```python
from build123d import *

# Parameters (mm, degrees)
F0_R     = 3.375
F0_R_2   = 2.6
F1_DEPTH = 13
F2_SIZE  = 3.5
F3_R     = 9
F4_DEPTH = 1.5


with BuildPart() as f1:
    # F0 (on Top) → F1 (new body)
    with BuildSketch(Plane.XY):
        with BuildLine():
            Line((-52.5, -62.5), (52.5, -62.5))
            ThreePointArc((52.5, -62.5), (59.571068, -59.571068), (62.5, -52.5))
            Line((62.5, -52.5), (62.5, 52.5))
            ThreePointArc((62.5, 52.5), (59.571068, 59.571068), (52.5, 62.5))
            Line((52.5, 62.5), (-52.5, 62.5))
            ThreePointArc((-52.5, 62.5), (-59.571068, 59.571068), (-62.5, 52.5))
            Line((-62.5, 52.5), (-62.5, -52.5))
            ThreePointArc((-62.5, -52.5), (-59.571068, -59.571068), (-52.5, -62.5))
        make_face()
        with Locations((-50, -50)):
            Circle(F0_R, mode=Mode.SUBTRACT)
        with Locations((-25, -50)):
            Circle(F0_R, mode=Mode.SUBTRACT)
        with Locations((0, -50)):
            Circle(F0_R, mode=Mode.SUBTRACT)
        with Locations((-50.3, -30)):
            Circle(F0_R_2, mode=Mode.SUBTRACT)
        with Locations((-25, -25)):
            Circle(F0_R, mode=Mode.SUBTRACT)
        with Locations((0, -25)):
            Circle(F0_R, mode=Mode.SUBTRACT)
        with Locations((25, -50)):
            Circle(F0_R, mode=Mode.SUBTRACT)
        with Locations((50, -50)):
            Circle(F0_R, mode=Mode.SUBTRACT)
        with Locations((25, -25)):
            Circle(F0_R, mode=Mode.SUBTRACT)
        with Locations((50.3, -30)):
            Circle(F0_R_2, mode=Mode.SUBTRACT)
        with Locations((-50, 0)):
            Circle(F0_R, mode=Mode.SUBTRACT)
        with Locations((-50.3, 30)):
            Circle(F0_R_2, mode=Mode.SUBTRACT)
        with Locations((-25, 0)):
            Circle(F0_R, mode=Mode.SUBTRACT)
        Circle(F0_R, mode=Mode.SUBTRACT)
        with Locations((-25, 25)):
            Circle(F0_R, mode=Mode.SUBTRACT)
        with Locations((0, 25)):
            Circle(F0_R, mode=Mode.SUBTRACT)
        with Locations((-50, 50)):
            Circle(F0_R, mode=Mode.SUBTRACT)
        with Locations((-25, 50)):
            Circle(F0_R, mode=Mode.SUBTRACT)
        with Locations((0, 50)):
            Circle(F0_R, mode=Mode.SUBTRACT)
        with Locations((25, 0)):
            Circle(F0_R, mode=Mode.SUBTRACT)
        with Locations((25, 25)):
            Circle(F0_R, mode=Mode.SUBTRACT)
        with Locations((50, 0)):
            Circle(F0_R, mode=Mode.SUBTRACT)
        with Locations((50.3, 30)):
            Circle(F0_R_2, mode=Mode.SUBTRACT)
        with Locations((25, 50)):
            Circle(F0_R, mode=Mode.SUBTRACT)
        with Locations((50, 50)):
            Circle(F0_R, mode=Mode.SUBTRACT)
    extrude(amount=F1_DEPTH)

    # F2
    f2_edges = [f1.edges().sort_by_distance(p)[0] for p in [
        (-52.9, 30, 13),
        (47.7, 30, 13),
        (47.7, -30, 13),
        (-52.9, -30, 13),
    ]]
    chamfer(f2_edges, length=F2_SIZE)

    # F3 (on face) → F4 (cut)
    with BuildSketch(Plane(origin=(0, 0, 0), x_dir=(1, 0, 0), z_dir=(0, 0, -1))):
        with Locations((0, 50)):
            Circle(F3_R)
        with Locations((0, 25)):
            Circle(F3_R)
        Circle(F3_R)
        with Locations((0, -25)):
            Circle(F3_R)
        with Locations((0, -50)):
            Circle(F3_R)
        with Locations((25, -25)):
            Circle(F3_R)
        with Locations((25, 0)):
            Circle(F3_R)
        with Locations((25, 25)):
            Circle(F3_R)
        with Locations((25, 50)):
            Circle(F3_R)
        with Locations((25, -50)):
            Circle(F3_R)
        with Locations((50, 0)):
            Circle(F3_R)
        with Locations((50, 50)):
            Circle(F3_R)
        with Locations((50, -50)):
            Circle(F3_R)
        with Locations((-25, 0)):
            Circle(F3_R)
        with Locations((-25, 25)):
            Circle(F3_R)
        with Locations((-25, -25)):
            Circle(F3_R)
        with Locations((-25, 50)):
            Circle(F3_R)
        with Locations((-25, -50)):
            Circle(F3_R)
        with Locations((-50, 0)):
            Circle(F3_R)
        with Locations((-50, 50)):
            Circle(F3_R)
        with Locations((-50, -50)):
            Circle(F3_R)
    extrude(amount=-F4_DEPTH, mode=Mode.SUBTRACT)


solid = f1.part
```
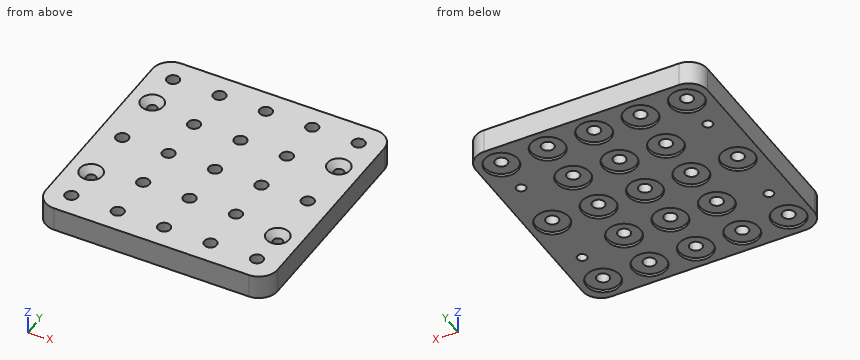
Geometry check sheet. Reference: the model listing, model coordinates, mm. Coordinates: 2 decimals unless noted, no trailing zeros. Order: outer loops, then holes, each group sorted by start corner. A loop starts at its lowest first (then second) coordinate and runs counter-clockwise, first axis right, second up. Notation, with made-up numbers: (-40, -14.75) - (12, -14.75) arc R17 cw to (12, 11.25) - close; hole circle Ø9 at (-5.5, 58.25). An arc over 180 degrees is marked (long way). Answer as a JSON object with one key per item and string values. Group by question number.
Item 1: Depth check by flat-ended pin: pin 1 Ø16 at (x, y) = (-25, -50) entering from +Z; pin 2 Ø4 at (x, y) = (-50.3, -30) entering from -Z; pin 3 Ø16 at (x, y) = (50, -50) entering from -Z. Enter the tip coordinate at first touch or a pass-through.
Item 2: Scan lines: probe 1 along Y at (x, z) = (25, 7) (3 decimals); probe 2 along X at (y, z) = (-50, 1.2); probe 3 along Y at (x, z) = (-50, 1.25). Record each from-to range of solid material in increasing order.
Item 3: Sectioned sample at A-A, the plane z = 5. Give the number of separate pieces and of enclosed holes in the cut face, and give its area (3 significant figures).
Item 4: Sectioned sample at B-B, the plane y = 30. Record the cut outline in (x, z).
Resolved:
{
 "1": {"pin 1": "z = 13", "pin 2": "through", "pin 3": "z = 1.5"},
 "2": {"probe 1": "-62.5 to -53.375, -46.625 to -28.375, -21.625 to -3.375, 3.375 to 21.625, 28.375 to 46.625, 53.375 to 62.5", "probe 2": "-62.5 to -59, -41 to -34, -16 to -9, 9 to 16, 34 to 41, 59 to 62.5", "probe 3": "-62.5 to -59, -41 to -32.58, -27.42 to -9, 9 to 27.42, 32.58 to 41, 59 to 62.5"},
 "3": {"separate pieces": "1", "enclosed holes": "25", "area": "14,700 mm^2"},
 "4": {"outline": "(-62.5, 0) - (-52.9, 0) - (-52.9, 9.5) - (-56.4, 13) - (-62.5, 13) - close; (-47.7, 0) - (-32.48, 0) - (-32.48, 1.5) - (-17.52, 1.5) - (-17.52, 0) - (-7.48, 0) - (-7.48, 1.5) - (7.48, 1.5) - (7.48, 0) - (17.52, 0) - (17.52, 1.5) - (32.48, 1.5) - (32.48, 0) - (47.7, 0) - (47.7, 9.5) - (44.2, 13) - (-44.2, 13) - (-47.7, 9.5) - close; (52.9, 0) - (62.5, 0) - (62.5, 13) - (56.4, 13) - (52.9, 9.5) - close"}
}
